Check sheet for the drawn part. Datum: minimum x, y, z corner. Units: mm. A direction names the side the tool comes from. Round coordinates to 2 decimals unless told otherwise and drop trailing zeros. Write each loop counter-clockwise with the first axis right and the second up, starting at its lowest first coordinate (ties: lowest second). Pieces come first, ordered by that corner, then holes. Notation, with made-up numbers: M 57.25,-10.5 L 76.25,-10.5 A35 ccw 76.25,23.5 Z; hole C -19,-18.5 d5. An arc over 180 degrees is marked long. One line per item, written item: value. Start each with the question number.
Item 1: Section check C-C, the plane y = 4.6. Record the cut outline in (x, z), then the cut area to 3 significant figures.
Item 2: Gauge pin test, flat ends, axial feed: pin 1 (2 mm diameter, centred on y = 4, z = 10, fed in from -X); pin 2 (3.5 mm diameter, centred on x = 6.5, z = 6.5, fed in from -Y); pin 3 (2 mm diameter, centred on y = 4.5, z = 8, fed in from +X); pin 4 (3 mm diameter, centred on y = 2.5, z = 2.5, fed in from +X). Record the tip position at first contact, or that the pin passes through.
Item 3: Section check A-A, the plane z = 6.5. Record the cut outline in (x, y).
Item 4: Tool access check on the marked faces 4 and 5. Record the directions out of +Z, -Z, +X, -X, +Y, -Y that give a thin tool (end or side, any length) a straight path to the whole face; none if there is none.
Item 5: Section check B-B, the plane x = 6.5. Record the cut outline in (y, z).
Item 6: Draft check along Z on the marked faces 1, 2 and 3. Enter one of: +Z half, -Z half, draft (parallel to the pull), parting line (faces both ways), or undercut.
Item 7: Section check D-D, the plane x = 10.75. Record the cut outline in (y, z), then the cut area to 3 significant figures.
Item 8: Thickness scan on probe 1 along Y at (x, z) = (9.25, 2); probe 2 along Z at (x, y) = (4, 3); probe 3 along X at (y, z) = (4.45, 4.25). Record the ranges inside material, lowest first. Write a range as from..to.
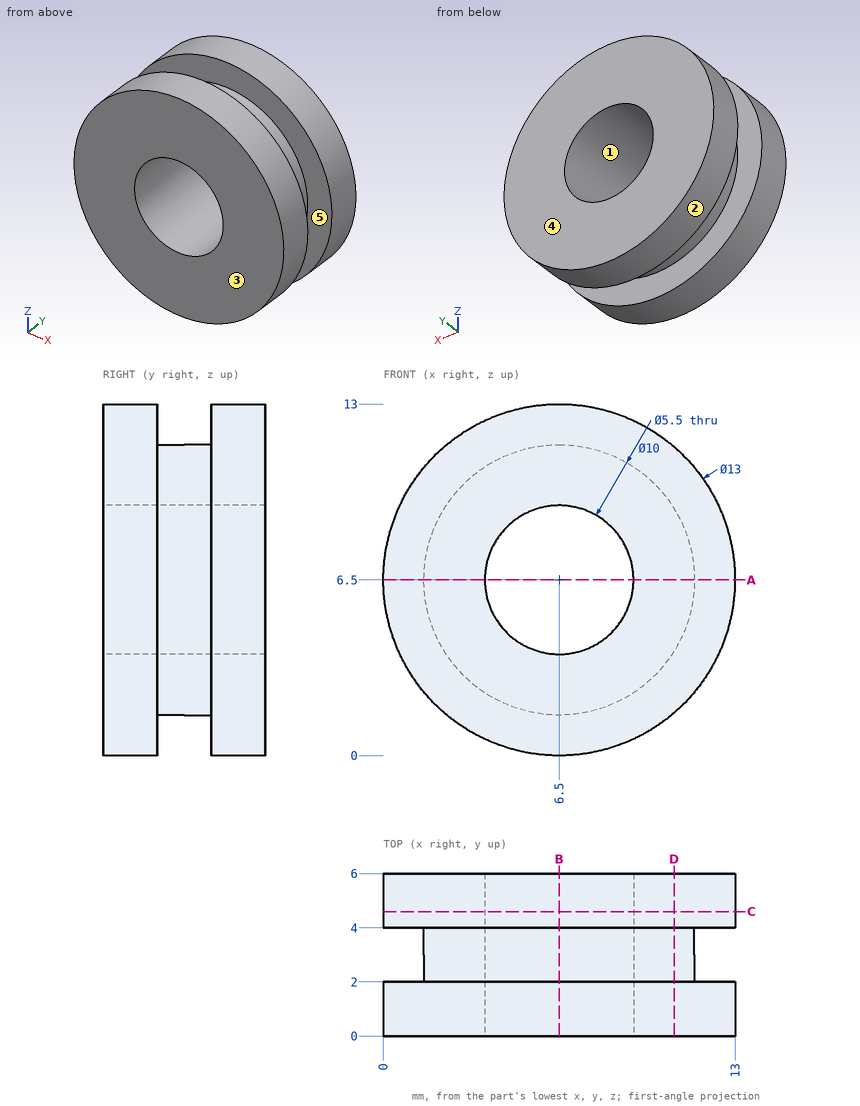
Response values:
1. outline: C 6.5,6.5 d13; hole C 6.5,6.5 d5.5
1. area: 109 mm2
2. pin 1: stops at x = 0.5
2. pin 2: passes through
2. pin 3: stops at x = 12.98
2. pin 4: stops at x = 12.46
3. outline: M 0,0 L 3.75,0 L 3.75,6 L 0,6 L 0,4 L 1.5,4 L 1.5,2 L 0,2 Z; M 9.25,0 L 13,0 L 13,2 L 11.5,2 L 11.5,4 L 13,4 L 13,6 L 9.25,6 Z
4. face 4: +Z, -Z, +X, -X, +Y
4. face 5: none
5. outline: M 0,0 L 2,0 L 2,1.5 L 4,1.5 L 4,0 L 6,0 L 6,3.75 L 0,3.75 Z; M 0,9.25 L 6,9.25 L 6,13 L 4,13 L 4,11.5 L 2,11.5 L 2,13 L 0,13 Z
6. face 1: undercut
6. face 2: parting line
6. face 3: draft
7. outline: M 0,1.58 L 2,1.58 L 2,3.87 L 4,3.87 L 4,1.58 L 6,1.58 L 6,11.42 L 4,11.42 L 4,9.13 L 2,9.13 L 2,11.42 L 0,11.42 Z
7. area: 49.9 mm2
8. probe 1: y = 0..2, 4..6
8. probe 2: z = 2.17..5.35, 7.65..10.83
8. probe 3: x = 0.4..4.92, 8.08..12.6
